Check sheet for the modelled part. Datum: model origin and axes. Units: mm. A direction names the side the tool comes from. Give positions to 0.01 mm unless a question says otherwise; leave off trailing zeros. Order: outer loops, then holes, each group sorted by start corner. A loop starts at its lowest first (then second) coordinate and runs counter-clockwise, first axis right, second up. Notation, with made-up numbers: (-10, 27) - (7, 27) arc R13 ccw to (7, 43) - close; hole circle Ø3 at (25, 43.5). An arc over 180 degrees is marked (long way). Answer in a Markdown table with one row per item.
from build123d import *

# Parameters (mm, degrees)
SKETCH_W     = 2000
SKETCH_H     = 900
PAD_DEPTH    = 50
SKETCH001_R  = 50
PAD001_DEPTH = 800


with BuildPart() as part:
    # Sketch → Pad (new body)
    with BuildSketch(Plane.XY):
        with Locations((1000, 450)):
            Rectangle(SKETCH_W, SKETCH_H)
    extrude(amount=PAD_DEPTH)

    # Sketch001 (on Face5 of Pad) → Pad001 (join)
    with BuildSketch(Plane(origin=(0, 0, 0), x_dir=(1, 0, 0), z_dir=(0, 0, -1))):
        with Locations((100, -100)):
            Circle(SKETCH001_R)
        with Locations((1900, -100)):
            Circle(SKETCH001_R)
        with Locations((1900, -800)):
            Circle(SKETCH001_R)
        with Locations((100, -800)):
            Circle(SKETCH001_R)
    extrude(amount=PAD001_DEPTH)


solid = part.part
(1) Cross-section at A-A, the plane x = 100. Record the cut outline in (y, z).
Geometry says:
| item | result |
|---|---|
| outline | (0, 0) - (50, 0) - (50, -800) - (150, -800) - (150, 0) - (750, 0) - (750, -800) - (850, -800) - (850, 0) - (900, 0) - (900, 50) - (0, 50) - close |
(2) Mould release check, pull along Y, two halves, no side actions. Record for faces 3 (the flat face through (99, 99, -800)), 4 (the cylindrical face through (1850.05, 797.8, -394.4)), 5 (the cylindrical face through (1850.05, 97.8, -394.4)), 6 (the flat face through (986, 900, 25)): pulls with the +Y half, pulls with the -Y half, needs draft (parallel to the pull), parting line crosses it, or undercut.
Geometry says:
| item | result |
|---|---|
| face 3 | needs draft |
| face 4 | undercut |
| face 5 | undercut |
| face 6 | pulls with the +Y half |
(3) Cross-section at C-C, the plane z = -365.5. Record the cut outline in (x, y).
Geometry says:
| item | result |
|---|---|
| outline | circle Ø100 at (100, 100); circle Ø100 at (100, 800); circle Ø100 at (1900, 100); circle Ø100 at (1900, 800) |
(4) Thickness scan on L1, parallel to Y at x = 97, z = -141; L2, parallel to Z at x = 725, y = 586; L3, parallel to X at y = 785.5, z = -496. Record the ranges inside material, lowest first.
Geometry says:
| item | result |
|---|---|
| L1 | 50.09 to 149.91, 750.09 to 849.91 |
| L2 | 0 to 50 |
| L3 | 52.15 to 147.85, 1852.15 to 1947.85 |
(5) Cross-section at D-D, the plane x = 531. Record the cut outline in (y, z).
Geometry says:
| item | result |
|---|---|
| outline | (0, 0) - (900, 0) - (900, 50) - (0, 50) - close |
(6) Cross-section at B-B, the plane y = 100. Record the cut outline in (x, z), then the cut area to 3 significant figures.
Geometry says:
| item | result |
|---|---|
| outline | (0, 0) - (50, 0) - (50, -800) - (150, -800) - (150, 0) - (1850, 0) - (1850, -800) - (1950, -800) - (1950, 0) - (2000, 0) - (2000, 50) - (0, 50) - close |
| area | 260,000 mm² |
(7) Access from +Z, -Z, +X, -X, +Y, -Y to the whole of each face (thin tool, end or side, straight path). Record for faces 1 (the cylindrical face through (60, 130, -394)), 2 (the flat face through (99, 799, -800)).
Geometry says:
| item | result |
|---|---|
| face 1 | -Z |
| face 2 | -Z, +X, -X, +Y, -Y |
(8) Gauge pin test, flat end, axial feed: P1, Ø4, axis at y = 785, z = -637, coming from the +X side. Record the tip position at first contact, or that the pin passes through.
Geometry says:
| item | result |
|---|---|
| P1 | x = 1948.28 |
